Design review of the part built by this model. Coordinates are the model's own, in mm. A direction names the side the tool comes from. Coordinates: 2 decimals unless noted, no trailing zeros. Write each loop counter-clockwise with the first axis right and the second up, starting at its lowest first coordinate (ties: lowest second). Pieces come first, ordered by that corner, then holes.
Q1. The part is to be moulded in two halves that separate along Y. For faces 4 (the flat face through (-839, -361.95, -433)), 5 (the flat face through (837, 387, -800.1)), 6 (the flat face through (-4, 438.15, -95)), say which applies: released by +Y, released by -Y, zero draft, split by the parting line, or undercut.
Q2. For pin 1 Ø15 at (y, z) = (-377, -311) entering from -X; pin 2 Ø8 at (x, y) = (43.5, 247.5) entering from -Z; pin 3 Ø3 at (y, z) = (-240, -96) entering from +X, all flat-tipped, find the tip position at first contact; note any pin that passes through.
Q3. Take a section at A-A, the plane x = -704.85. Write out the cut boundary in (y, z), plus the area to 3 significant figures.
Q4. Take a section at B-B, the plane y = -137. Write out the cut boundary in (x, z).
Q5. For faces 1 (the flat face through (-863.6, 2, -93)), 2 (the flat face through (-839, -336.55, -446)), 3 (the flat face through (787.4, -387, -446)), list the 3-axis set-ups (+Z, -Z, +X, -X, +Y, -Y) from which the entire face can be reached by the end or side of a thin tool; tool diameter is ignored.
Q6. For L1, parallel to X at y = 374, z = -19; L2, parallel to X at y = 399, z = -758.5; L3, parallel to Y at x = 736.6, z = -18, list the stretches that pass through material, from the lowest coordinate up.
Q7. Take a section at D-D, the plane x = -83.5. Write out the cut boundary in (y, z), plus the area to 3 significant figures.
Q8. Take a section at C-C, the plane z = -217.5. State how many separate pieces and enclosed holes the cut face has, plus the area to 3 significant figures.
from build123d import *

# Parameters (mm, degrees)
F1_W        = 1828.8
F1_H        = 927.1
F2_DEPTH    = 25.4
F0_W        = 1778
F0_H        = 876.3
F3_DEPTH    = 101.6
F4_W        = 101.6
F4_H        = 101.6
F5_DEPTH    = 698.5
F6_T        = 25.4
F6_T3_DEPTH = 927.1
F6_T5_DEPTH = 1828.8
F7_R        = 31.75
F8_DEPTH    = 25.4
F9_SIZE     = 12.7
F10_R       = 5.08
F11_SIZE    = 5.08


# Not quite as in the source:
# - a shell that OpenCascade refuses in one call is made with other operations: the cavity is built on its own and cut out


with BuildPart() as f2:
    # F1 (on Top) → F2 (new body)
    with BuildSketch(Plane.XY):
        Rectangle(F1_W, F1_H)
    extrude(amount=-F2_DEPTH)

    # F0 (on Top) → F3 (join)
    with BuildSketch(Plane.XY):
        Rectangle(F0_W, F0_H)
    extrude(amount=-F3_DEPTH)

    # F4 (on face) → F5 (join)
    with BuildSketch(Plane(origin=(0, 0, -101.6), x_dir=(1, 0, 0), z_dir=(0, 0, -1))):
        with Locations((-838.2, 387.35)):
            Rectangle(F4_W, F4_H)
        with Locations((-838.2, -387.35)):
            Rectangle(F4_W, F4_H)
        with Locations((838.2, 387.35)):
            Rectangle(F4_W, F4_H)
        with Locations((838.2, -387.35)):
            Rectangle(F4_W, F4_H)
    extrude(amount=F5_DEPTH)

    # F6: shell of thickness 25.4, made by hand


with BuildPart() as f6_core1:
    # F6_t2: copy of F2
    add(f2.part)

    # the walls: a layer under each face that stays
    f6_faces = [f6_core1.faces().sort_by_distance(p)[0] for p in [
        (0, 463.55, -12.7),
        (628.65, -452.1043209877, -25.4),
        (762, 438.15, -80.7357142857),
        (-838.2, 387.35, -800.1),
        (-838.2, 336.55, -450.85),
        (-787.4, 387.35, -450.85),
        (-838.2, -336.55, -450.85),
        (-838.2, -387.35, -800.1),
        (-787.4, -387.35, -450.85),
        (787.4, -387.35, -450.85),
        (838.2, -387.35, -800.1),
        (838.2, -336.55, -450.85),
        (838.2, 336.55, -450.85),
        (787.4, 387.35, -450.85),
        (838.2, 387.35, -800.1),
        (889, -375.5571428571, -744.7642857143),
        (-762, -438.15, -80.7357142857),
        (-889, 375.5571428571, -744.7642857143),
        (0, -463.55, -12.7),
        (0, 0, 0),
        (-914.4, 0, -12.7),
        (914.4, 0, -12.7),
    ]]
    thicken(f6_faces, amount=-F6_T, mode=Mode.SUBTRACT)

    # F6_s4 → F6_t3 (cut)
    with BuildSketch(Plane.XZ.offset(-463.55)):
        Polygon((-889.254, -25.654), (-889, 0), (-863.6, 0), (-863.6, -25.4), align=None)
        Polygon((889.254, -25.654), (889, 0), (863.6, 0), (863.6, -25.4), align=None)
    extrude(amount=F6_T3_DEPTH, mode=Mode.SUBTRACT)

    # F6_s6 → F6_t5 (cut)
    with BuildSketch(Plane.YZ.offset(-914.4)):
        Polygon((-438.404, -25.654), (-438.15, 0), (-412.75, 0), (-412.75, -25.4), align=None)
        Polygon((438.404, -25.654), (438.15, 0), (412.75, 0), (412.75, -25.4), align=None)
    extrude(amount=F6_T5_DEPTH, mode=Mode.SUBTRACT)


with BuildPart() as f2_1:
    add(f2.part)

    # what is left inside the walls is the cavity
    f6_cavity = [f6_core1.part.solids().sort_by_distance(p)[0] for p in [
        (0, -137.583333, -25.654),
    ]]
    add(f6_cavity, mode=Mode.SUBTRACT)

    # F7 (on face) → F8 (cut)
    with BuildSketch(Plane.XY):
        with Locations((-704.85, 374.65)):
            Circle(F7_R)
        with Locations((736.6, 374.65)):
            Circle(F7_R)
    extrude(amount=-F8_DEPTH, mode=Mode.SUBTRACT)

    # F9
    f9_edges = [f2_1.edges().sort_by_distance(p)[0] for p in [
        (0, -463.55, 0),
        (-914.4, 0, 0),
        (0, 463.55, 0),
        (914.4, 0, 0),
    ]]
    chamfer(f9_edges, length=F9_SIZE)

    # F10
    f10_edges = [f2_1.edges().sort_by_distance(p)[0] for p in [
        (-889, -438.15, -412.75),
        (-787.4, -438.15, -450.85),
        (-889, -336.55, -450.85),
        (-787.4, -336.55, -450.85),
        (787.4, -438.15, -450.85),
        (889, -438.15, -412.75),
        (787.4, -336.55, -450.85),
        (889, -336.55, -450.85),
        (889, 336.55, -450.85),
        (787.4, 336.55, -450.85),
        (889, 438.15, -412.75),
        (787.4, 438.15, -450.85),
        (-889, 438.15, -412.75),
        (-787.4, 438.15, -450.85),
        (-889, 336.55, -450.85),
        (-787.4, 336.55, -450.85),
    ]]
    fillet(f10_edges, radius=F10_R)

    # F11
    f11_edges = [f2_1.edges().sort_by_distance(p)[0] for p in [
        (-889, 0, -101.6),
        (0, -438.15, -101.6),
        (889, 0, -101.6),
        (0, 438.15, -101.6),
    ]]
    chamfer(f11_edges, length=F11_SIZE)


solid = f2_1.part
Responses:
1. face 4: undercut
1. face 5: zero draft
1. face 6: released by +Y
2. pin 1: stops at x = -889
2. pin 2: stops at z = -25.4
2. pin 3: stops at x = 889
3. outline: (-463.55, -25.4) - (-438.15, -25.4) - (-438.15, -96.52) - (-433.07, -101.6) - (-412.75, -101.6) - (-412.75, -25.4) - (342.9, -25.4) - (342.9, 0) - (-450.85, 0) - (-463.55, -12.7) - close; (406.4, -25.4) - (412.75, -25.4) - (412.75, -101.6) - (433.07, -101.6) - (438.15, -96.52) - (438.15, -25.4) - (463.55, -25.4) - (463.55, -12.7) - (450.85, 0) - (406.4, 0) - close
3. area: 25,600 mm2
4. outline: (-914.4, -25.4) - (-889, -25.4) - (-889, -96.52) - (-883.92, -101.6) - (-863.6, -101.6) - (-863.6, -25.4) - (863.6, -25.4) - (863.6, -101.6) - (883.92, -101.6) - (889, -96.52) - (889, -25.4) - (914.4, -25.4) - (914.4, -12.7) - (901.7, 0) - (-901.7, 0) - (-914.4, -12.7) - close
5. face 1: none
5. face 2: -Z, +X, -X
5. face 3: -Z, +Y, -Y
6. L1: x = -914.4 to -736.59, -673.11 to 704.86, 768.34 to 914.4
6. L2: x = -889 to -863.6, -812.8 to -787.4, 787.4 to 812.8, 863.6 to 889
6. L3: y = -463.55 to 342.9, 406.4 to 463.55
7. outline: (-463.55, -25.4) - (-438.15, -25.4) - (-438.15, -96.52) - (-433.07, -101.6) - (-412.75, -101.6) - (-412.75, -25.4) - (412.75, -25.4) - (412.75, -101.6) - (433.07, -101.6) - (438.15, -96.52) - (438.15, -25.4) - (463.55, -25.4) - (463.55, -12.7) - (450.85, 0) - (-450.85, 0) - (-463.55, -12.7) - close
7. area: 27,200 mm2
8. separate pieces: 4
8. enclosed holes: 4
8. area: 30,900 mm2
